from build123d import *

# Parameters (mm, degrees)
SALIENTE_EXTRUIR1_DEPTH = 2


with BuildPart() as part:
    # Croquis1 → Saliente-Extruir1 (new body)
    with BuildSketch(Plane.XY):
        with BuildLine():
            Line((-1.909727018, 12.353256361), (-1.639945169, 15.320856699))
            Line((-1.639945169, 15.320856699), (1.639945169, 15.320856699))
            Line((1.639945169, 15.320856699), (1.909727018, 12.353256361))
            ThreePointArc((1.909727018, 12.353256361), (3.86271243, 11.888206454), (5.716060295, 11.116503709))
            Line((5.716060295, 11.116503709), (7.678630109, 13.358769022))
            Line((7.678630109, 13.358769022), (10.332117131, 11.430897853))
            Line((10.332117131, 11.430897853), (8.806063519, 8.871484955))
            ThreePointArc((8.806063519, 8.871484955), (10.11271243, 7.347315654), (11.158506856, 5.633624476))
            Line((11.158506856, 5.633624476), (14.064229672, 6.294085627))
            Line((14.064229672, 6.294085627), (15.077771526, 3.174724549))
            Line((15.077771526, 3.174724549), (12.338783063, 2.001107827))
            ThreePointArc((12.338783063, 2.001107827), (12.5, 0), (12.338783063, -2.001107827))
            Line((12.338783063, -2.001107827), (15.077771526, -3.174724549))
            Line((15.077771526, -3.174724549), (14.064229672, -6.294085627))
            Line((14.064229672, -6.294085627), (11.158506856, -5.633624476))
            ThreePointArc((11.158506856, -5.633624476), (10.11271243, -7.347315654), (8.806063519, -8.871484955))
            Line((8.806063519, -8.871484955), (10.332117131, -11.430897853))
            Line((10.332117131, -11.430897853), (7.678630109, -13.358769022))
            Line((7.678630109, -13.358769022), (5.716060295, -11.116503709))
            ThreePointArc((5.716060295, -11.116503709), (3.86271243, -11.888206454), (1.909727018, -12.353256361))
            Line((1.909727018, -12.353256361), (1.639945169, -15.320856699))
            Line((1.639945169, -15.320856699), (-1.639945169, -15.320856699))
            Line((-1.639945169, -15.320856699), (-1.909727018, -12.353256361))
            ThreePointArc((-1.909727018, -12.353256361), (-3.86271243, -11.888206454), (-5.716060295, -11.116503709))
            Line((-5.716060295, -11.116503709), (-7.678630109, -13.358769022))
            Line((-7.678630109, -13.358769022), (-10.332117131, -11.430897853))
            Line((-10.332117131, -11.430897853), (-8.806063519, -8.871484955))
            ThreePointArc((-8.806063519, -8.871484955), (-10.11271243, -7.347315654), (-11.158506856, -5.633624476))
            Line((-11.158506856, -5.633624476), (-14.064229672, -6.294085627))
            Line((-14.064229672, -6.294085627), (-15.077771526, -3.174724549))
            Line((-15.077771526, -3.174724549), (-12.338783063, -2.001107827))
            ThreePointArc((-12.338783063, -2.001107827), (-12.5, 0), (-12.338783063, 2.001107827))
            Line((-12.338783063, 2.001107827), (-15.077771526, 3.174724549))
            Line((-15.077771526, 3.174724549), (-14.064229672, 6.294085627))
            Line((-14.064229672, 6.294085627), (-11.158506856, 5.633624476))
            ThreePointArc((-11.158506856, 5.633624476), (-10.11271243, 7.347315654), (-8.806063519, 8.871484955))
            Line((-8.806063519, 8.871484955), (-10.332117131, 11.430897853))
            Line((-10.332117131, 11.430897853), (-7.678630109, 13.358769022))
            Line((-7.678630109, 13.358769022), (-5.716060295, 11.116503709))
            ThreePointArc((-5.716060295, 11.116503709), (-3.86271243, 11.888206454), (-1.909727018, 12.353256361))
        make_face()
    extrude(amount=SALIENTE_EXTRUIR1_DEPTH)


solid = part.part
Can you work these out from the model? Positions are in its coordinate system, mm. A direction names the side the tool comes from. Round coordinates to 2 decimals unless told otherwise and drop trailing zeros. Write each loop counter-clockwise with the first axis right and the second up, starting at its lowest first coordinate (ties: lowest second). Pieces come first, ordered by that corner, then holes. Notation, with made-up numbers: (-37.5, -25) -> (5.5, -25) arc R16 cw to (5.5, -6) -> close; hole circle Ø5 at (-16.5, 34.5). An arc over 180 degrees is marked (long way). One line per question, with ' | ' between items. Start each with the question number.
1) I'm going to push flat-ended pins straight in: P1, Ø1, axis at x = -6, z = 1, coming from the -Y side; P2, Ø1, axis at x = -5.5, z = 0.5, coming from the +Y side; P3, Ø1, axis at x = -6.5, z = 1, coming from the -Y side. Where does each tip first touch, or does it pass through?
2) On a 3-axis mill with a long thin cutter (end or side, diameter ignored), from which of +Z, -Z, +X, -X, +Y, -Y can I reach the whole of each face in a straight line? I mean faces 1 (the flat face through (1.777, -13.816, 0.986)), 2 (the cylindrical face through (-10.096, -7.37, 0.986)), 3 (the flat face through (-9.6, -10.2, 1)), 4 (the flat face through (9.558, -10.133, 0.986)). Say none if no direction works.
3) Suppose I cut it at D-D on y = 7. Write out the boundary of the cut face in (x, z), then the cut area to 3 significant figures.
4) If we mould it in two halves opening along X, with no side actions, what happens to faces 5 (the flat face through (-6.71, 12.25, 0.99)), 6 (the flat face through (-9, -12.4, 1)), 7 (the flat face through (13.727, 2.596, 0.986))? For each: released by +X, released by -X, zero draft, split by the parting line, or undercut.
5) I need wall thicknesses on line 1 (X direction, y = -11.5, z = 0.3); line 2 (X direction, y = 13, z = 0.45); line 3 (Y direction, x = 9, z = 0.4). Which ranges of each line are inside material? Lowest first, please. Write a range as [from, to].
6) Suppose I cut it at A-A on y = -13. Write out the boundary of the cut face in (x, z).
7) Suppose I cut it at C-C on x = -3. Write out the boundary of the cut face in (y, z), then the cut area to 3 significant figures.
8) Suppose I cut it at B-B on y = 12. Write out the boundary of the cut face in (x, z).
Return value:
1) P1: stops at y = -12.01 | P2: stops at y = 11.46 | P3: stops at y = -12.58
2) face 1: +Z, -Z, -Y | face 2: +Z, -Z | face 3: +Z, -Z, -X | face 4: +Z, -Z, +X
3) outline: (-10.36, 0) -> (10.36, 0) -> (10.36, 2) -> (-10.36, 2) -> close | area: 41.4 mm2
4) face 5: undercut | face 6: released by -X | face 7: released by +X
5) line 1: x = [-10.24, -6.05], [-4.9, 4.9], [6.05, 10.24] | line 2: x = [-8.17, -7.36], [-1.85, 1.85], [7.36, 8.17] | line 3: y = [-12.4, -9.2], [-8.67, 8.67], [9.2, 12.4]
6) outline: (-8.17, 0) -> (-7.36, 0) -> (-7.36, 2) -> (-8.17, 2) -> close; (-1.85, 0) -> (1.85, 0) -> (1.85, 2) -> (-1.85, 2) -> close; (7.36, 0) -> (8.17, 0) -> (8.17, 2) -> (7.36, 2) -> close
7) outline: (-12.13, 0) -> (12.13, 0) -> (12.13, 2) -> (-12.13, 2) -> close | area: 48.5 mm2
8) outline: (-9.55, 0) -> (-6.49, 0) -> (-6.49, 2) -> (-9.55, 2) -> close; (-3.5, 0) -> (3.5, 0) -> (3.5, 2) -> (-3.5, 2) -> close; (6.49, 0) -> (9.55, 0) -> (9.55, 2) -> (6.49, 2) -> close
